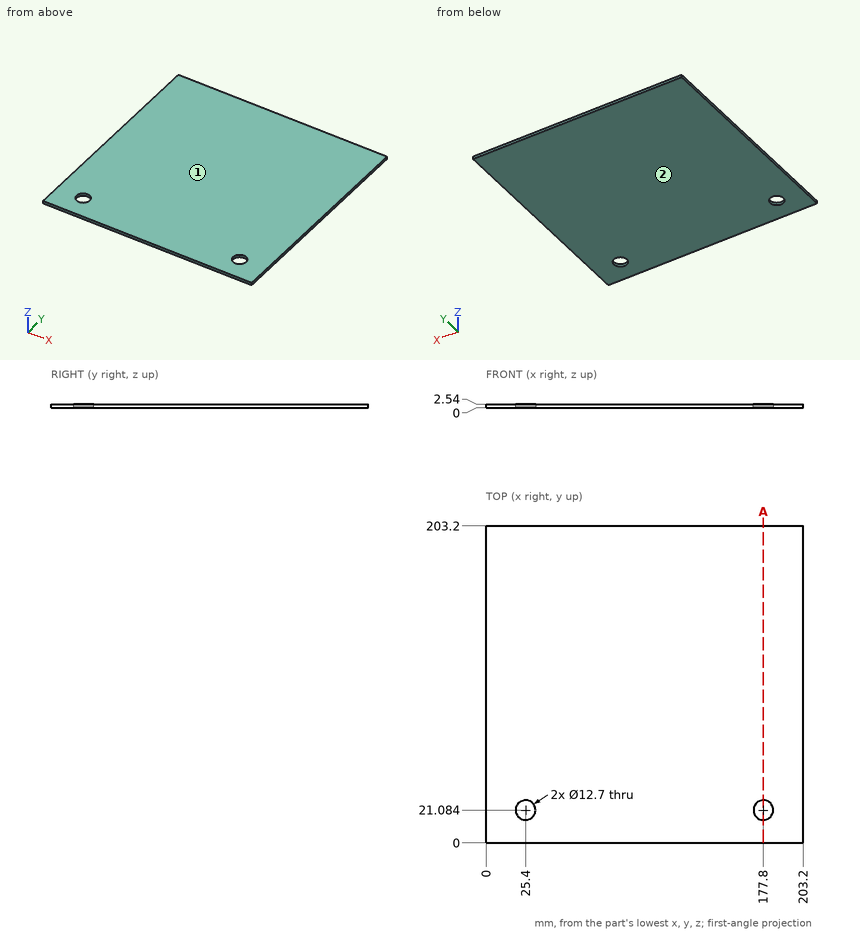
Answer from the drawing. Dimensions are ordinates in mm from the lowest x, y and z of the part. Round coordinates to 2 decimals unless told otherwise and drop trailing zeros. Loops run counter-clockwise (first coordinate to the right, second up) from the corner with the lowest first, then second, coordinate; pieces in that order, holes last. Notation, with made-up numbers: (-37.75, 41.25) - (-8.75, 41.25) arc R16 ccw to (-8.75, 52.25) - close; hole circle Ø2 at (-14, 49.25). An arc over 180 degrees is marked (long way). One line per item, written item: value.
Q1. Find section A-A on x = 177.8. Give the vertices of the cut face in (y, z).
Check values:
outline: (0, 0) - (14.73, 0) - (14.73, 2.54) - (0, 2.54) - close; (27.43, 0) - (203.2, 0) - (203.2, 2.54) - (27.43, 2.54) - close
Q2. The mould has two halves that part along Z. Classify the marked faces 1 and 2: +Z half, -Z half, draft (parallel to the pull), parting line (faces both ways), or undercut.
Check values:
face 1: +Z half
face 2: -Z half
Q3. Straight lines are drawn through the part: probe 1 along X at (y, z) = (21, 2.15); probe 2 along Y at (x, z) = (25.4, 0.6); probe 3 along X at (y, z) = (26.5, 1.7) (1 decimal). For each, find the intervals that lie inside material, in ascending order.
Check values:
probe 1: 0 to 19.05, 31.75 to 171.45, 184.15 to 203.2
probe 2: 0 to 14.73, 27.43 to 203.2
probe 3: 0 to 22.1, 28.7 to 174.5, 181.1 to 203.2
